The model under review builds one solid part; all positions refer to its coordinate system, in mm. Give positions to 0.01 mm unless a question says otherwise; leave off trailing zeros. Write each loop counter-clockwise with the first axis right and the second up, starting at its lowest first coordinate (ties: lowest second). Pieces come first, ordered by that corner, then holes. Notation, with made-up numbers: (21.25, 61.25) -> (73.25, 61.25) arc R18 cw to (73.25, 67.25) -> close; hole circle Ø4 at (-28, 3). An arc over 180 degrees is marked (long way). Use CSV: the item, a comma, the result in double quotes.
```python
from build123d import *

# Parameters (mm, degrees)
ESBO_O1_W                = 40
ESBO_O1_H                = 30
RESSALTO_EXTRUS_O1_DEPTH = 4
CORTE_EXTRUS_O1_REACH    = 27.318
ESBO_O2_R                = 1.5


with BuildPart() as part:
    # Esboço1 → Ressalto-extrusão1 (new body)
    with BuildSketch(Plane.XY):
        Rectangle(ESBO_O1_W, ESBO_O1_H)
    extrude(amount=RESSALTO_EXTRUS_O1_DEPTH)

    # Esboço2 → Corte-extrusão1 (cut, up to next)
    with BuildSketch(Plane.XY.offset(4), mode=Mode.PRIVATE) as corte_extrus_o1_sk1:
        Circle(ESBO_O2_R)
    corte_extrus_o1_tool1 = extrude(corte_extrus_o1_sk1.sketch, amount=-CORTE_EXTRUS_O1_REACH, mode=Mode.PRIVATE) & part.part
    # Esboço2 → Corte-extrusão1 (cut, up to next)
    with BuildSketch(Plane.XY.offset(4), mode=Mode.PRIVATE) as corte_extrus_o1_sk2:
        with Locations((-10, 0)):
            Circle(ESBO_O2_R)
    corte_extrus_o1_tool2 = extrude(corte_extrus_o1_sk2.sketch, amount=-CORTE_EXTRUS_O1_REACH, mode=Mode.PRIVATE) & part.part
    # Esboço2 → Corte-extrusão1 (cut, up to next)
    with BuildSketch(Plane.XY.offset(4), mode=Mode.PRIVATE) as corte_extrus_o1_sk3:
        with Locations((10, 0)):
            Circle(ESBO_O2_R)
    corte_extrus_o1_tool3 = extrude(corte_extrus_o1_sk3.sketch, amount=-CORTE_EXTRUS_O1_REACH, mode=Mode.PRIVATE) & part.part
    add(corte_extrus_o1_tool1.solids().sort_by_distance((0, 0, 4))[0], mode=Mode.SUBTRACT)
    add(corte_extrus_o1_tool2.solids().sort_by_distance((-10, 0, 4))[0], mode=Mode.SUBTRACT)
    add(corte_extrus_o1_tool3.solids().sort_by_distance((10, 0, 4))[0], mode=Mode.SUBTRACT)


solid = part.part
```
Q1. To check wall thickness, follow probe 1 along Y at (x, z) = (-10, 3.25); probe 2 along Y at (x, z) = (1, 3.75). State the ranges of each line that lie inside material, in increasing order.
Derived:
probe 1,"y = -15 to -1.5, 1.5 to 15"
probe 2,"y = -15 to -1.12, 1.12 to 15"
Q2. The part is to be moulded in two halves that separate along X. For faces 1 (the cylindrical face through (8.5, 0.07, 2.03)), 2 (the flat face through (0, 15, 2)), 3 (the cylindrical face through (-11.5, 0.07, 2.03)), 4 (the flat face through (20, 0, 2)), say which applies: pulls with the +X half, pulls with the -X half, needs draft (parallel to the pull), parting line crosses it, or undercut.
Derived:
face 1,"undercut"
face 2,"needs draft"
face 3,"undercut"
face 4,"pulls with the +X half"
Q3. Consider section A-A (x = -10). Write out the cut boundary in (y, z), then the cut area to 3 significant figures.
Derived:
outline,"(-15, 0) -> (-1.5, 0) -> (-1.5, 4) -> (-15, 4) -> close; (1.5, 0) -> (15, 0) -> (15, 4) -> (1.5, 4) -> close"
area,"108 mm2"
Q4. Consider section B-B (y = -0.75). Write out the cut boundary in (x, z).
Derived:
outline,"(-20, 0) -> (-11.3, 0) -> (-11.3, 4) -> (-20, 4) -> close; (-8.7, 0) -> (-1.3, 0) -> (-1.3, 4) -> (-8.7, 4) -> close; (1.3, 0) -> (8.7, 0) -> (8.7, 4) -> (1.3, 4) -> close; (11.3, 0) -> (20, 0) -> (20, 4) -> (11.3, 4) -> close"
Q5. Insertion check: pin 1 (1.8 mm diameter, centred on x = 10, y = 0, fed in from -Z); pin 2 (12 mm diameter, centred on x = 3, y = 3.5, fed in from -Z). Each pin has a flat end and moves straight along its axis. Give the tip position at first contact, or say it passes through.
Derived:
pin 1,"passes through"
pin 2,"stops at z = 0"
Q6. Consider section D-D (x = 1). Write out the cut boundary in (y, z).
Derived:
outline,"(-15, 0) -> (-1.12, 0) -> (-1.12, 4) -> (-15, 4) -> close; (1.12, 0) -> (15, 0) -> (15, 4) -> (1.12, 4) -> close"
Q7. Consider section C-C (z = 1). Write out the cut boundary in (x, y), then the cut area to 3 significant figures.
Derived:
outline,"(-20, -15) -> (20, -15) -> (20, 15) -> (-20, 15) -> close; hole circle Ø3 at (-10, 0); hole circle Ø3 at (0, 0); hole circle Ø3 at (10, 0)"
area,"1,180 mm2"
